from build123d import *

# Parameters (mm, degrees)
SKETCH_1_W          = 34.5
SKETCH_1_H          = 5
EXTRUDE_1_DEPTH     = 2
SKETCH_1_9_R        = 0.75
CUT_EXTRUDE_1_DEPTH = 18.54458606
SKETCH_1_10_W       = 2
SKETCH_1_10_H       = 5
SKETCH_1_10_W_2     = 3
SKETCH_1_10_H_2     = 2.5
EXTRUDE_2_DEPTH     = 4.6
EXTRUDE_START       = 4.6
SKETCH_1_12_W       = 3
SKETCH_1_12_H       = 3
SKETCH_1_12_R       = 0.6
SKETCH_1_12_H_2     = 5
EXTRUDE_3_DEPTH     = 1.5


with BuildPart() as part:
    # 草图1 → 凸台-拉伸1 (new body)
    with BuildSketch(Plane.XY):
        Rectangle(SKETCH_1_W, SKETCH_1_H)
    extrude(amount=EXTRUDE_1_DEPTH)

    # 草图1<9> → 切除-拉伸1 (cut, through all)
    with BuildSketch(Plane.XY):
        with Locations((-16.25, 0)):
            Circle(SKETCH_1_9_R)
        with Locations((-13.75, 0)):
            Circle(SKETCH_1_9_R)
        with Locations((-6.25, 0)):
            Circle(SKETCH_1_9_R)
        with Locations((-3.75, 0)):
            Circle(SKETCH_1_9_R)
        with Locations((3.75, 0)):
            Circle(SKETCH_1_9_R)
        with Locations((6.25, 0)):
            Circle(SKETCH_1_9_R)
        with Locations((13.75, 0)):
            Circle(SKETCH_1_9_R)
        with Locations((16.25, 0)):
            Circle(SKETCH_1_9_R)
    extrude(amount=CUT_EXTRUDE_1_DEPTH, mode=Mode.SUBTRACT)

    # 草图1<10> → 凸台-拉伸2 (add)
    with BuildSketch(Plane.XY):
        with Locations((-18.25, 0)):
            Rectangle(SKETCH_1_10_W, SKETCH_1_10_H)
        with Locations((18.25, 0)):
            Rectangle(SKETCH_1_10_W, SKETCH_1_10_H)
        with Locations((0, 1.25)):
            Rectangle(SKETCH_1_10_W_2, SKETCH_1_10_H_2)
        with Locations((0, -1.25)):
            Rectangle(SKETCH_1_10_W_2, SKETCH_1_10_H_2)
    extrude(amount=EXTRUDE_2_DEPTH)

    # 草图1<12> → 凸台-拉伸3 (add)
    # profile 1 of 4: a face of its own
    with BuildSketch(Plane.XY.offset(EXTRUDE_START)):
        with Locations((0, 4)):
            Rectangle(SKETCH_1_12_W, SKETCH_1_12_H)
        with Locations((0, 4)):
            Circle(SKETCH_1_12_R, mode=Mode.SUBTRACT)
    # profile 2 of 4: a face of its own
    with BuildSketch(Plane.XY.offset(EXTRUDE_START)):
        with Locations((-20.75, 0)):
            Rectangle(SKETCH_1_12_W, SKETCH_1_12_H_2)
        with Locations((-20.75, 0)):
            Circle(SKETCH_1_12_R, mode=Mode.SUBTRACT)
    # profile 3 of 4: a face of its own
    with BuildSketch(Plane.XY.offset(EXTRUDE_START)):
        with Locations((0, -4)):
            Rectangle(SKETCH_1_12_W, SKETCH_1_12_H)
        with Locations((0, -4)):
            Circle(SKETCH_1_12_R, mode=Mode.SUBTRACT)
    # profile 4 of 4: a face of its own
    with BuildSketch(Plane.XY.offset(EXTRUDE_START)):
        with Locations((20.75, 0)):
            Rectangle(SKETCH_1_12_W, SKETCH_1_12_H_2)
        with Locations((20.75, 0)):
            Circle(SKETCH_1_12_R, mode=Mode.SUBTRACT)
    extrude(amount=-EXTRUDE_3_DEPTH)


solid = part.part
Could you check a few things on this model? Use its own coordinates, in mm. A direction names the side the tool comes from. Give positions to 0.01 mm unless a question says otherwise; leave off trailing zeros. Write each loop counter-clockwise with the first axis right and the second up, starting at its lowest first coordinate (ties: lowest second). Pieces come first, ordered by that corner, then holes. Notation, with made-up numbers: (42.5, -20.75) - (98.5, -20.75) arc R31 ccw to (98.5, 11.25) - close; hole circle Ø2 at (10.5, -36.5). An arc over 180 degrees is marked (long way). Use CSV: the item, a comma, the result in double quotes. Start each with the question number.
Item 1: I'm going to push flat-ended pins straight in: pin 1 (1 mm diameter, centred on x = 0, y = 4, fed in from +Z); pin 2 (2 mm diameter, centred on x = -16.5, z = 1.5, fed in from -Y); pin 3 (1 mm diameter, centred on y = 1.5, z = 3, fed in from +X); pin 4 (1.4 mm diameter, centred on x = 5, z = 2, fed in from +Y). Where does each tip first touch, or does it pass through?
Item 2: I want a section at B-B, the plane z = 0.75. Give the number of separate pieces and of enclosed holes in the cut face, then the cut area to 3 significant figures.
Item 3: I want a section at C-C, the plane y = -1.25. Please give me the cut outline in (x, z), then the cut area to 3 significant figures.
Item 4: If we mould it in two halves opening along Y, with no side actions, what happens to faces 5 (the face through (3, 0, 1)), 6 (the face through (-22.25, 0, 4)), 7 (the face through (0, -2.5, 2))? For each: pulls with the +Y half, pulls with the -Y half, needs draft (parallel to the pull), parting line crosses it, or undercut.
Item 5: For faces 1 (the face through (-1.5, 0, 4)), 2 (the face through (20, -1, 3.1)), 3 (the face through (-7, 0, 1)), 4 (the face through (-21, -1, 3.1)), which set-ups out of +Z, -Z, +X, -X, +Y, -Y let a thin tool reach every point of the face, with its end or its side?
Item 6: If I drill on line 1 along Y through (x, z) = (0, 3.9); line 2 along Y through (x, z) = (-13.75, 1.4); line 3 along X through (y, z) = (0.25, 3.55), over which ranges is the centre line in solid material (lowest first)?
Item 7: I want a section at D-D, the plane z = 2.6. Please give me the cut outline in (x, y), then the cut area to 3 significant figures.
Item 8: I want a section at A-A, the plane x = 13.75. Please give me the cut outline in (y, z), then the cut area to 3 significant figures.
Findings:
1,pin 1,"passes through"
1,pin 2,"stops at y = -2.5"
1,pin 3,"stops at x = 22.25"
1,pin 4,"stops at y = 2.5"
2,separate pieces,"1"
2,enclosed holes,"8"
2,area,"178 mm2"
3,outline,"(-22.25, 3.1) - (-19.25, 3.1) - (-19.25, 0) - (19.25, 0) - (19.25, 3.1) - (22.25, 3.1) - (22.25, 4.6) - (17.25, 4.6) - (17.25, 2) - (1.5, 2) - (1.5, 4.6) - (-1.5, 4.6) - (-1.5, 2) - (-17.25, 2) - (-17.25, 4.6) - (-22.25, 4.6) - close"
3,area,"104 mm2"
4,face 5,"undercut"
4,face 6,"needs draft"
4,face 7,"pulls with the -Y half"
5,face 1,"+Z, +Y, -Y"
5,face 2,"-Z, +X, +Y, -Y"
5,face 3,"+Z, -Z"
5,face 4,"-Z, -X, +Y, -Y"
6,line 1,"y = -5.5 to -4.6, -3.4 to 3.4, 4.6 to 5.5"
6,line 2,"y = -2.5 to -0.75, 0.75 to 2.5"
6,line 3,"x = -22.25 to -21.3, -20.2 to -17.25, -1.5 to 1.5, 17.25 to 20.2, 21.3 to 22.25"
7,outline,"(-19.25, -2.5) - (-17.25, -2.5) - (-17.25, 2.5) - (-19.25, 2.5) - close; (-1.5, -2.5) - (1.5, -2.5) - (1.5, 2.5) - (-1.5, 2.5) - close; (17.25, -2.5) - (19.25, -2.5) - (19.25, 2.5) - (17.25, 2.5) - close"
7,area,"35.0 mm2"
8,outline,"(-2.5, 0) - (-0.75, 0) - (-0.75, 2) - (-2.5, 2) - close; (0.75, 0) - (2.5, 0) - (2.5, 2) - (0.75, 2) - close"
8,area,"7.00 mm2"
